Build history of the part. All positions in model axes, mm. Face numbers are marked on the shaded views. A direction names the side the tool comes from. Round coordinates to 2 decimals unless told otherwise and drop trailing zeros. Write each loop counter-clockwise with the first axis right and the second up, starting at its lowest first coordinate (ties: lowest second). Pieces come first, ordered by that corner, then holes. Notation, with made-up numbers: (-17.5, -15.5) -> (29.5, -15.5) arc R15 cw to (29.5, -9.5) -> close; hole circle Ø7 at (38.5, -15). An arc over 180 degrees is marked (long way). Return JSON: item names as keys, results as strings.
from build123d import *

# Parameters (mm, degrees)
SKETCH074_W     = 42.3
SKETCH074_H     = 3
SKETCH075_W     = 42.3
SKETCH075_H     = 3
SKETCH076_R     = 1.5
PAD030_DEPTH    = 5
SKETCH033_R     = 1.5000289281
SKETCH033_R_2   = 1.500028928
PAD031_DEPTH    = 5
SKETCH078_R     = 2.75
SKETCH078_R_2   = 3.175
POCKET020_DEPTH = 5
SKETCH084_W     = 140
SKETCH084_H     = 3.0000000001
SKETCH084_H_2   = 3
PAD034_DEPTH    = 2
FILLET005_R     = 1.4
SKETCH088_W     = 15.725
SKETCH088_H     = 15.725
SKETCH088_R     = 3.175
PAD036_DEPTH    = 2
FILLET006_R     = 1.3


with BuildPart() as part:
    # Sketch074 (on Face1 of Binder022) → AdditiveLoft005 section 0
    with BuildSketch(Plane.YZ.offset(-204)):
        with Locations((0, -67.2022145348)):
            Rectangle(SKETCH074_W, SKETCH074_H)
    # Sketch075 (on Face1 of Binder023) → AdditiveLoft005 section 1
    with BuildSketch(Plane(origin=(-64, 0, 0), x_dir=(0, -1, 0), z_dir=(-1, 0, 0))):
        with Locations((0, -67.2022145348)):
            Rectangle(SKETCH075_W, SKETCH075_H)
    loft()

    # Sketch076 (on Face1 of Binder023) → Pad030 (new body)
    with BuildSketch(Plane(origin=(-64, 0, 0), x_dir=(0, -1, 0), z_dir=(-1, 0, 0))):
        with BuildLine():
            Line((-12.15, -71.7022145347), (-12.15, -68.7022145348))
            Line((-12.15, -68.7022145348), (-21.15, -68.7022145348))
            Line((-21.15, -68.7022145348), (-21.15, -71.7022145347))
            ThreePointArc((-21.15, -71.7022145347), (-16.65, -76.2022145528), (-12.15, -71.7022145347))
        make_face()
        with Locations((-16.65, -71.7022145528)):
            Circle(SKETCH076_R, mode=Mode.SUBTRACT)
        with BuildLine():
            Line((12.15, -71.7022145347), (12.15, -68.7022145348))
            Line((12.15, -68.7022145348), (21.15, -68.7022145348))
            Line((21.15, -68.7022145348), (21.15, -71.7022145347))
            ThreePointArc((12.15, -71.7022145347), (16.65, -76.20221451), (21.15, -71.7022145347))
        make_face()
        with Locations((16.65, -71.70221451)):
            Circle(SKETCH076_R, mode=Mode.SUBTRACT)
    extrude(amount=PAD030_DEPTH)

    # Sketch033 (on Face1 of Binder022) → Pad031 (join)
    with BuildSketch(Plane.YZ.offset(-204)):
        with BuildLine():
            Line((-21.1499999998, -71.7022145347), (-21.15, -68.7022145348))
            Line((-21.15, -68.7022145348), (-12.15, -68.7022145348))
            Line((-12.15, -68.7022145348), (-12.1500000002, -71.7022145347))
            ThreePointArc((-21.1499999998, -71.7022145347), (-16.65, -76.2022525186), (-12.1500000002, -71.7022145347))
        make_face()
        with Locations((-16.65, -71.7022434628)):
            Circle(SKETCH033_R, mode=Mode.SUBTRACT)
        with BuildLine():
            Line((12.1500000002, -71.7022145347), (12.15, -68.7022145348))
            Line((12.15, -68.7022145348), (21.15, -68.7022145348))
            Line((21.15, -68.7022145348), (21.1499999998, -71.7022145347))
            ThreePointArc((12.1500000002, -71.7022145347), (16.65, -76.2022525185), (21.1499999998, -71.7022145347))
        make_face()
        with Locations((16.65, -71.7022434628)):
            Circle(SKETCH033_R_2, mode=Mode.SUBTRACT)
    extrude(amount=PAD031_DEPTH)

    # Sketch078 (on Face5 of Pad031) → Pocket020 (cut)
    with BuildSketch(Plane(origin=(0, 0, -68.7022145348), x_dir=(1, 0, 0), z_dir=(0, 0, -1))):
        with Locations((-149.5, 15.5)):
            Circle(SKETCH078_R)
        with Locations((-118.5, 15.5)):
            Circle(SKETCH078_R)
        with Locations((-118.5, -15.5)):
            Circle(SKETCH078_R)
        with Locations((-149.5, -15.5)):
            Circle(SKETCH078_R)
        with Locations((-134, 0)):
            Circle(SKETCH078_R_2)
        with BuildLine():
            ThreePointArc((-159.5, 12.75), (-156.75, 15.5), (-159.5, 18.25))
            Line((-159.5, 18.25), (-184.5, 18.25))
            ThreePointArc((-184.5, 18.25), (-187.25, 15.5), (-184.5, 12.75))
            Line((-184.5, 12.75), (-159.5, 12.75))
        make_face()
        with BuildLine():
            ThreePointArc((-159.5, -18.25), (-156.75, -15.5), (-159.5, -12.75))
            Line((-159.5, -12.75), (-184.5, -12.75))
            ThreePointArc((-184.5, -12.75), (-187.25, -15.5), (-184.5, -18.25))
            Line((-184.5, -18.25), (-159.5, -18.25))
        make_face()
        with BuildLine():
            ThreePointArc((-108.5, -12.75), (-111.25, -15.5), (-108.5, -18.25))
            Line((-108.5, -18.25), (-83.5, -18.25))
            ThreePointArc((-83.5, -18.25), (-80.75, -15.5), (-83.5, -12.75))
            Line((-83.5, -12.75), (-108.5, -12.75))
        make_face()
        with BuildLine():
            ThreePointArc((-108.5, 18.25), (-111.25, 15.5), (-108.5, 12.75))
            Line((-108.5, 12.75), (-83.5, 12.75))
            ThreePointArc((-83.5, 12.75), (-80.75, 15.5), (-83.5, 18.25))
            Line((-83.5, 18.25), (-108.5, 18.25))
        make_face()
        with BuildLine():
            ThreePointArc((-128.5, 12.75), (-125.75, 15.5), (-128.5, 18.25))
            Line((-128.5, 18.25), (-139.5, 18.25))
            ThreePointArc((-139.5, 18.25), (-142.25, 15.5), (-139.5, 12.75))
            Line((-139.5, 12.75), (-128.5, 12.75))
        make_face()
        with BuildLine():
            ThreePointArc((-139.5, -12.75), (-142.25, -15.5), (-139.5, -18.25))
            Line((-139.5, -18.25), (-128.5, -18.25))
            ThreePointArc((-128.5, -18.25), (-125.75, -15.5), (-128.5, -12.75))
            Line((-128.5, -12.75), (-139.5, -12.75))
        make_face()
    extrude(amount=-POCKET020_DEPTH, mode=Mode.SUBTRACT)

    # Sketch084 (on Face5 of Pocket020) → Pad034 (join)
    with BuildSketch(Plane(origin=(0, 0, -68.7022145348), x_dir=(1, 0, 0), z_dir=(0, 0, -1))):
        with Locations((-134, 7.9625)):
            Rectangle(SKETCH084_W, SKETCH084_H)
        with Locations((-134, -7.9625)):
            Rectangle(SKETCH084_W, SKETCH084_H_2)
    extrude(amount=PAD034_DEPTH)

    # Fillet005
    fillet005_edges = [part.edges().sort_by_distance(p)[0] for p in [
        (-134, -9.4625, -70.702215),
        (-64, -7.9625, -70.702215),
        (-134, -6.4625, -70.702215),
        (-204, -7.9625, -70.702215),
        (-134, 6.4625, -70.702215),
        (-204, 7.9625, -70.702215),
        (-134, 9.4625, -70.702215),
        (-64, 7.9625, -70.702215),
    ]]
    fillet(fillet005_edges, radius=FILLET005_R)

    # Sketch088 (on Face8 of Fillet005) → Pad036 (join)
    with BuildSketch(Plane(origin=(0, 0, -68.7022145348), x_dir=(1, 0, 0), z_dir=(0, 0, -1))):
        with Locations((-134, 0)):
            Rectangle(SKETCH088_W, SKETCH088_H)
        with Locations((-134, 0)):
            Circle(SKETCH088_R, mode=Mode.SUBTRACT)
    extrude(amount=PAD036_DEPTH)

    # Fillet006
    fillet006_edges = [part.edges().sort_by_distance(p)[0] for p in [
        (-126.1375, 0, -70.702215),
        (-141.8625, 0, -70.702215),
    ]]
    fillet(fillet006_edges, radius=FILLET006_R)


solid = part.part
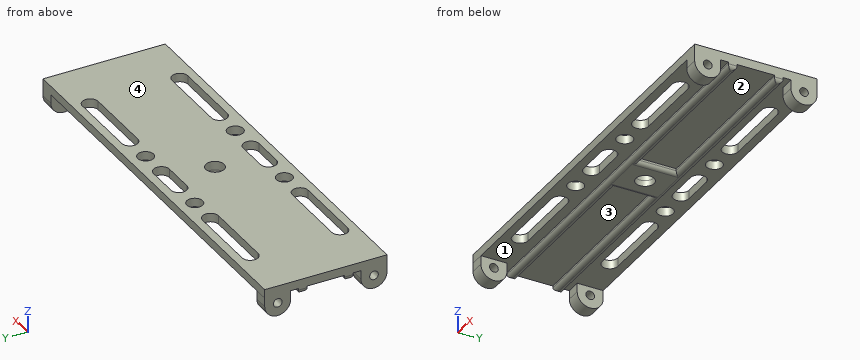
Q1. Saw through at C-C on x = -118.5. List the corners of the cut face in (y, z).
Verdict:
{"outline": "(-21.15, -68.7) -> (-18.25, -68.7) -> (-18.25, -65.7) -> (-21.15, -65.7) -> close; (-12.75, -68.7) -> (-9.46, -68.7) -> (-9.46, -69.3) arc R1.4 ccw to (-8.06, -70.7) -> (-7.86, -70.7) arc R1.4 ccw to (-6.46, -69.3) -> (-6.46, -68.7) -> (6.46, -68.7) -> (6.46, -69.3) arc R1.4 ccw to (7.86, -70.7) -> (8.06, -70.7) arc R1.4 ccw to (9.46, -69.3) -> (9.46, -68.7) -> (12.75, -68.7) -> (12.75, -65.7) -> (-12.75, -65.7) -> close; (18.25, -68.7) -> (21.15, -68.7) -> (21.15, -65.7) -> (18.25, -65.7) -> close"}
Q2. Two-plate mould, pull along X, no slides. Class the marked faces 1 and 2: +X half, -X half, draft (parallel to the pull), parting line (faces both ways), or undercut.
Verdict:
{"face 1": "undercut", "face 2": "draft"}
Q3. Wall check: L1, parallel to X at y = -15.5, z = -67.5; L2, parallel to Y at x = -134, z = -66.35 (3 decimals); L3, parallel to Y at x = -149.5, z = -67.4. Give the ranges that are in metal, low to high.
Verdict:
{"L1": "x = -204 to -187.25, -156.75 to -152.25, -146.75 to -142.25, -125.75 to -121.25, -115.75 to -111.25, -80.75 to -64", "L2": "y = -21.15 to -18.25, -12.75 to -3.175, 3.175 to 12.75, 18.25 to 21.15", "L3": "y = -21.15 to -18.25, -12.75 to 12.75, 18.25 to 21.15"}
Q4. 3-axis set-ups, long thin cutter, end or side, ignore diameter. For the marked faces 3 and 4: which of +Z, -Z, +X, -X, +Y, -Y reach the whole face in a straight line?
Verdict:
{"face 3": "-Z, -X", "face 4": "+Z, +X, -X, +Y, -Y"}
Q5. Saw through at D-D on x = -194.5. List the corners of the cut face in (y, z), then the cut area to 3 significant figures.
Verdict:
{"outline": "(-21.15, -68.7) -> (-9.46, -68.7) -> (-9.46, -69.3) arc R1.4 ccw to (-8.06, -70.7) -> (-7.86, -70.7) arc R1.4 ccw to (-6.46, -69.3) -> (-6.46, -68.7) -> (6.46, -68.7) -> (6.46, -69.3) arc R1.4 ccw to (7.86, -70.7) -> (8.06, -70.7) arc R1.4 ccw to (9.46, -69.3) -> (9.46, -68.7) -> (21.15, -68.7) -> (21.15, -65.7) -> (-21.15, -65.7) -> close", "area": "137 mm²"}
Q6. Saw through at A-A on x = -134. Count the separate pieces of the cut face and the enclosed holes in it, then the cut area to 3 significant figures.
Verdict:
{"separate pieces": "4", "enclosed holes": "0", "area": "99.2 mm²"}
Q7. Pin check, flat tips, straight feed: pin 1 Ø8 at (x, y) = (-142, 3.5) entering from -Z; pin 2 Ø5 at (x, y) = (-176.5, -1.5) entering from -Z; pin 3 Ø2 at (x, z) = (-185, -71) entering from +Y. Stop position of each tip, or through.
Verdict:
{"pin 1": "stops at z = -70.7", "pin 2": "stops at z = -68.7", "pin 3": "stops at y = 9.28"}
